Job drawing, mm, ordinate dimensions from the low corner. One solid piece. Coordinates: 2 decimals unless noted, no trailing zeros. Order: outer loops, then holes, each group sorted by start corner. A loop starts at its lowest first (then second) coordinate and runs counter-clockwise, first axis right, second up. Notation, with made-up numbers: (-4, 51.5) -> (5, 51.5) arc R20 cw to (5, 61.5) -> close; hole circle Ø7 at (0, -14.75). An arc over 180 degrees is marked (long way). Use CSV: the item, a comma, the result in double quotes. Start each with the question number.
(1) Cut at B-B on x = 25. Give the number of separate pieces and of enclosed holes in the cut face, plus the area to 3 significant figures.
(2) Probe L1, parallel to Y at x = 4.5, z = 34.5; L2, parallel to Z at x = 26, y = 10.5; L3, parallel to Z at x = 8.75, y = 6.25. List the from-to ranges inside material, lowest first.
(3) Pin check, flat tips, straight feed: pin 1 Ø4 at (x, z) = (25, 41.25) entering from -Y; pin 2 Ø1.5 at (x, y) = (10.5, 8.5) entering from -Z; pin 3 Ø3 at (x, y) = (33.5, 7) entering from -Z; pin 4 Ø4 at (y, z) = (6.5, 39) entering from -X. Stop position of each tip, or through.
(4) Cut at A-A on y = 12.75. Write the cut outline in (x, z), plus the area to 3 significant figures.
(5) Pull direction Z, two halves, no side cores. Call the marked faces 1 and 2: pulls with the +Z half, pulls with the -Z half, needs draft (parallel to the pull), parting line crosses it, or undercut.
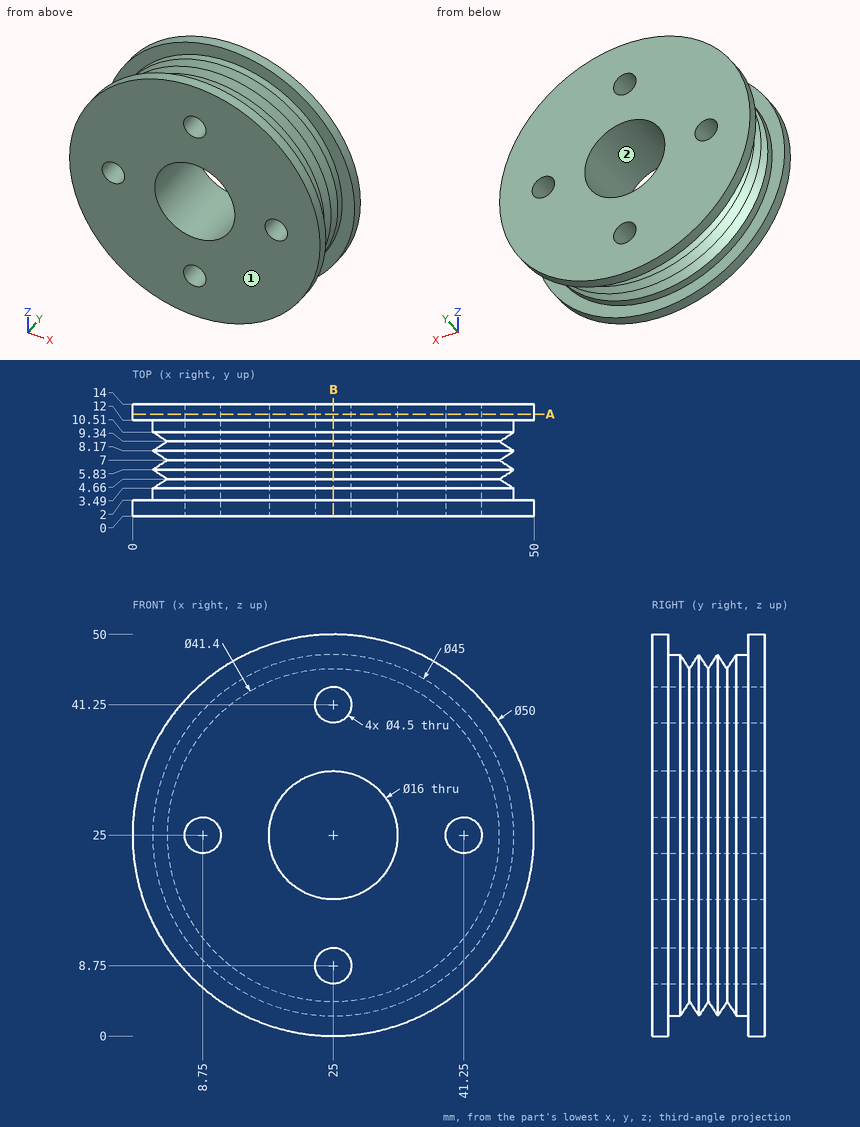
Outcome:
1,separate pieces,"4"
1,enclosed holes,"0"
1,area,"287 mm2"
2,L1,"0 to 2, 12 to 14"
2,L2,"2.54 to 6.73, 10.77 to 17.06, 32.94 to 39.23, 43.27 to 47.46"
2,L3,"10.39 to 22.75, 27.25 to 39.61"
3,pin 1,"through"
3,pin 2,"z = 7.25"
3,pin 3,"z = 3.81"
3,pin 4,"x = 6.04"
4,outline,"circle Ø50 at (25, 25); hole circle Ø4.5 at (8.75, 25); hole circle Ø16 at (25, 25); hole circle Ø4.5 at (25, 8.75); hole circle Ø4.5 at (25, 41.25); hole circle Ø4.5 at (41.25, 25)"
4,area,"1,700 mm2"
5,face 1,"needs draft"
5,face 2,"undercut"
